Work out the finished part from the listing and answer in its coordinate system (mm). Face numbers are marked on the shaded views. Give positions to 0.01 mm unless a question says otherwise; leave off trailing zeros. Loops run counter-clockwise (first coordinate to the right, second up) from the corner with the lowest first, then second, coordinate; pieces in that order, holes last. Notation, with made-up numbers: M 7.25,-2.75 L 21.25,-2.75 A21 cw 21.25,4.25 Z; hole C 21,19.25 d7. An arc over 180 degrees is marked long. Answer as a JSON object with one key per item and string values. Group by question number.
Autodesk Inventor part; units mm, degrees
ref_plane "YZ Plane" through (0, 0, 0) normal (1, 0, 0) x (0, 1, 0)
ref_plane "XZ Plane" through (0, 0, 0) normal (0, 1, 0) x (-1, 0, 0)
ref_plane "XY Plane" through (0, 0, 0) normal (0, 0, 1) x (1, 0, 0)
sketch "Sketch1" plane through (0, 0, 0) normal (0, 0, 1) x (1, 0, 0)
  line L0 (-25, 27) -> (-25, 0)
  line L1 (-25, 0) -> (-25.75, 0)
  line L2 (-25.75, 0) -> (-25.75, 6)
  line L3 (-25.75, 6) -> (-27, 6)
  line L4 (-27, 6) -> (-27, 24.1865)
  line L5 (-37.5, 30) -> (-26, 30)
  line L6 (-26, 30) -> (-26, 27)
  line L7 (-26, 27) -> (-25, 27)
  line L8 (0, -6) -> (0, 36)
  line L9 (-37.5, 30) -> (-37.5, 27)
  line L10 (-37.5, 27) -> (-27, 24.1865)
  point P0 (0, 0)
  dimension "d0" = 25.75
  dimension "neck_ir" = 25
  dimension "d5" = 6
  dimension "d15" = 27
  dimension "d16" = 3
  dimension "d17" = 37.5
  dimension "d18" = 26
  dimension "d19" = 15
  dimension "d20" = 3
  dimension "d21" = 30
revolve "Revolution1" add sketch "Sketch1" angle 360 about axis through (0, -10, 0) along (0, 1, 0)
equation "\"oring_diameter\" = 4"
properties part number "neckForStorage" material "Brass"
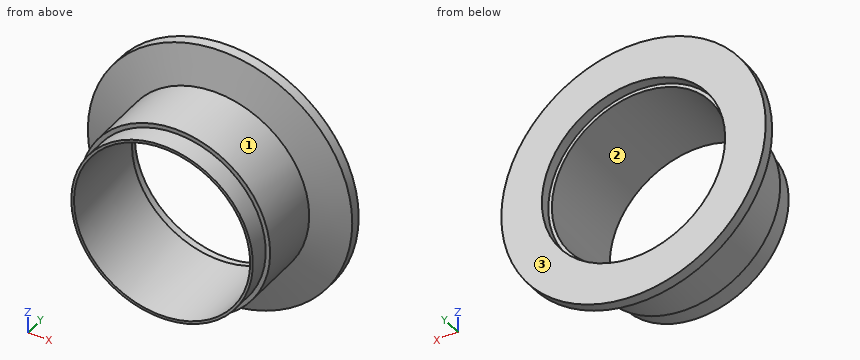
Item 1: A cutting plane is placed at D-D (y = 2.75). Determine the outline of the cut face in (x, z), and give its area (3 significant figures).
Item 2: For a pull along Z with two mould halves and no side action, classify the marked faces 1, 2 and 3 as pulls with the +Z half, pulls with the -Z half, needs draft (parallel to the pull), parting line crosses it, or undercut.
Item 3: A cutting plane is placed at B-B (z = 0). Determine the outline of the cut face in (x, y).
Item 4: A cutting plane is placed at C-C (y = 19.25). Determine the outline of the cut face in (x, z), and give its area (3 significant figures).
Item 5: Given pin 1 Ø6 at (x, y) = (7.5, 14.5) entering from -Z; pin 2 Ø3 at (x, z) = (11.5, 28.5) entering from -Y; pin 3 Ø12 at (x, y) = (6, 25.5) entering from +Z, each flat-ended and moving along its own axis, determine where each tip first touches the part or whether it passes through.
Item 6: Find the intervals of material crossed by probe 1 along Z at (x, y) = (0, 28.1); probe 2 along Z at (x, y) = (0, 6.75); probe 3 along Y at (x, z) = (27, 2), in increasing order. Write a range as [from, to].
Item 7: A cutting plane is placed at A-A (x = 0). Determine the outline of the cut face in (y, z).
The answers:
{
 "1": {"outline": "C 0,0 d51.5; hole C 0,0 d50", "area": "120 mm^2"},
 "2": {"face 1": "parting line crosses it", "face 2": "undercut", "face 3": "needs draft"},
 "3": {"outline": "M -37.5,27 L -27,24.19 L -27,6 L -25.75,6 L -25.75,0 L -25,0 L -25,27 L -26,27 L -26,30 L -37.5,30 Z; M 25,0 L 25.75,0 L 25.75,6 L 27,6 L 27,24.19 L 37.5,27 L 37.5,30 L 26,30 L 26,27 L 25,27 Z"},
 "4": {"outline": "C 0,0 d54; hole C 0,0 d50", "area": "327 mm^2"},
 "5": {"pin 1": "stops at z = -26.62", "pin 2": "stops at y = 24.78", "pin 3": "stops at z = 37.5"},
 "6": {"probe 1": "z = [-37.5, -26], [26, 37.5]", "probe 2": "z = [-27, -25], [25, 27]", "probe 3": "y = [24.21, 30]"},
 "7": {"outline": "M 0,-25.75 L 6,-25.75 L 6,-27 L 24.19,-27 L 27,-37.5 L 30,-37.5 L 30,-26 L 27,-26 L 27,-25 L 0,-25 Z; M 0,25 L 27,25 L 27,26 L 30,26 L 30,37.5 L 27,37.5 L 24.19,27 L 6,27 L 6,25.75 L 0,25.75 Z"}
}
